Check sheet for the modelled part. Datum: model origin and axes. Units: mm. Face numbers are marked on the shaded views. A direction names the side the tool comes from. Give positions to 0.01 mm unless a question says otherwise; leave off trailing zeros. Write each loop counter-clockwise with the first axis right and the second up, starting at its lowest first coordinate (ties: lowest second). Pieces come first, ordered by that corner, then holes. Notation, with made-up numbers: (87, 13) -> (125, 13) arc R13 cw to (125, 20) -> close; hole circle Ø10 at (78.25, 32). An arc over 180 degrees is marked (long way). Use a Markdown table: item, result. Add a question column.
1. Gauge pin test, flat ends, axial feed: P1, Ø3.5, axis at x = 13.42, y = 7.75, coming from the -Z side; P2, Ø10, axis at x = -11.5, z = 6, coming from the -Y side; P3, Ø3, axis at x = -5, y = -13.5, coming from the +Z side; P4, Ø5, axis at y = -9.5, z = 60, coming from the -X side. Record the tip position at first contact, or that the pin passes through.
2. Scan lines: probe 1 along X at (y, z) = (-7, 50); probe 2 along X at (y, z) = (7, 51); probe 3 along Z at (x, y) = (4, 13.5). Record each from-to range of solid material in increasing order. Write a range as [from, to].
3. Cross-section at B-B (z = 9). Enter the section's corners in (x, y), then the cut area to 3 significant figures.
4. Release check for a two-part mould opening along Y. For the marked faces 1, 2 and 3 record: released by +Y, released by -Y, zero draft, split by the parting line, or undercut.
5. Set-up check for the marked faces 4, 5 and 6: record each of +Z, -Z, +X, -X, +Y, -Y from which the full face is reachable in a straight line by a thin tool's end or side.
6. Cross-section at C-C (z = 43.5). Enter the section's corners in (x, y), then the cut area to 3 significant figures.
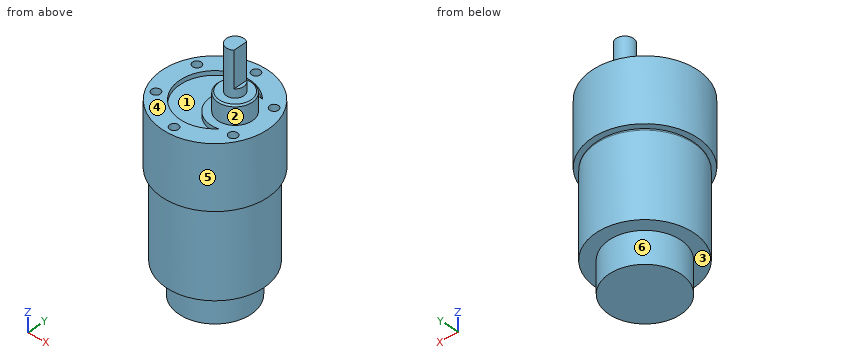
from build123d import *

# Parameters (mm, degrees)
SKETCH1_R           = 17
BOSS_EXTRUDE1_DEPTH = 30
FILLET1_R           = 1
SKETCH2_R           = 18.4
BOSS_EXTRUDE2_DEPTH = 22
SKETCH3_R           = 1.5
CUT_EXTRUDE1_DEPTH  = 3
SKETCH4_R           = 6
BOSS_EXTRUDE3_DEPTH = 6.5
CHAMFER1_SIZE       = 0.5
SKETCH5_R           = 3
BOSS_EXTRUDE4_DEPTH = 15.5
CUT_EXTRUDE3_DEPTH  = 1.5
SKETCH7_R           = 12.5
BOSS_EXTRUDE5_DEPTH = 11
CUT_EXTRUDE4_DEPTH  = 12.5


with BuildPart() as part:
    # Sketch1 → Boss-Extrude1 (new body)
    with BuildSketch(Plane.XY):
        Circle(SKETCH1_R)
    extrude(amount=BOSS_EXTRUDE1_DEPTH)

    # Fillet1
    fillet1_edges = [part.edges().sort_by_distance(p)[0] for p in [
        (-17, 0, 30),
    ]]
    fillet(fillet1_edges, radius=FILLET1_R)

    # Sketch2 → Boss-Extrude2 (add)
    with BuildSketch(Plane.XY.offset(30)):
        Circle(SKETCH2_R)
    extrude(amount=BOSS_EXTRUDE2_DEPTH)

    # Sketch3 → Cut-Extrude1 (cut)
    with BuildSketch(Plane.XY.offset(52)):
        with Locations((0, 15.5)):
            Circle(SKETCH3_R)
        with Locations((13.423393759, 7.75)):
            Circle(SKETCH3_R)
        with Locations((13.423393759, -7.75)):
            Circle(SKETCH3_R)
        with Locations((0, -15.5)):
            Circle(SKETCH3_R)
        with Locations((-13.423393759, -7.75)):
            Circle(SKETCH3_R)
        with Locations((-13.423393759, 7.75)):
            Circle(SKETCH3_R)
    extrude(amount=-CUT_EXTRUDE1_DEPTH, mode=Mode.SUBTRACT)

    # Sketch4 → Boss-Extrude3 (add)
    with BuildSketch(Plane.XY.offset(52)):
        with Locations((7, 0)):
            Circle(SKETCH4_R)
    extrude(amount=BOSS_EXTRUDE3_DEPTH)

    # Chamfer1
    chamfer1_edges = [part.edges().sort_by_distance(p)[0] for p in [
        (1, 0, 58.5),
    ]]
    chamfer(chamfer1_edges, length=CHAMFER1_SIZE)

    # Sketch5 → Boss-Extrude4 (add)
    with BuildSketch(Plane.XY.offset(58.5)):
        with Locations((7, 0)):
            Circle(SKETCH5_R)
    extrude(amount=BOSS_EXTRUDE4_DEPTH)

    # Sketch6 → Cut-Extrude3 (cut)
    with BuildSketch(Plane.XY.offset(52)):
        with BuildLine():
            ThreePointArc((8.868134735, -8.359715213), (-1.565907181, 0), (8.868134735, 8.359715213))
            ThreePointArc((8.868134735, 8.359715213), (-12.187233161, 0), (8.868134735, -8.359715213))
        make_face()
    extrude(amount=-CUT_EXTRUDE3_DEPTH, mode=Mode.SUBTRACT)

    # Sketch7 → Boss-Extrude5 (add)
    with BuildSketch(Plane(origin=(0, 0, 0), x_dir=(-1, 0, 0), z_dir=(0, 0, -1))):
        Circle(SKETCH7_R)
    extrude(amount=BOSS_EXTRUDE5_DEPTH)

    # Sketch8 → Cut-Extrude4 (cut)
    with BuildSketch(Plane.XY.offset(74)):
        with BuildLine():
            Line((8.779351905, 2.415348174), (8.779351905, -2.415348174))
            ThreePointArc((8.779351905, -2.415348174), (10, 0), (8.779351905, 2.415348174))
        make_face()
    extrude(amount=-CUT_EXTRUDE4_DEPTH, mode=Mode.SUBTRACT)


solid = part.part
Worked answers:
| question | item | result |
|---|---|---|
| 1 | P1 | stops at z = 0 |
| 1 | P2 | stops at y = -15.71 |
| 1 | P3 | stops at z = 52 |
| 1 | P4 | passes through |
| 2 | probe 1 | x = [-17.02, -14.72], [-12.12, 12.12], [14.72, 17.02] |
| 2 | probe 2 | x = [-17.02, -14.72], [-12.12, -9.98], [2.06, 12.12], [14.72, 17.02] |
| 2 | probe 3 | z = [0, 52] |
| 3 | outline | circle Ø34 at (0, 0) |
| 3 | area | 908 mm² |
| 4 | face 1 | undercut |
| 4 | face 2 | split by the parting line |
| 4 | face 3 | zero draft |
| 5 | face 4 | +Z |
| 5 | face 5 | +Z, -Z |
| 5 | face 6 | -Z |
| 6 | outline | circle Ø36.8 at (0, 0) |
| 6 | area | 1,060 mm² |
